from build123d import *

# Parameters (mm, degrees)
F0_R         = 7.935
F1_DEPTH     = 20
F2_DEPTH     = 12.7
F4_DEPTH     = 12.7
F6_T1_DEPTH  = 77.0257979591
F6_T3_DEPTH  = 76.8715237662
F6_T5_DEPTH  = 231
F6_T8_ANGLE  = 60.7302478015
F6_T12_DEPTH = 65.5200608313
F6_T17_DEPTH = 65.5200608313
F6_T20_ANGLE = 60.7302478015
F6_T22_ANGLE = 60.7302478015
F6_T26_DEPTH = 65.5200608313
F6_T31_DEPTH = 65.5200608313
F6_T34_ANGLE = 60.7302478015


# Not quite as in the source:
# - a fillet or chamfer that OpenCascade refuses, or shapes differently, is made with other operations: its cross-section is extruded or revolved along the edge and cut away or added


with BuildPart() as f1:
    # F0 (on Top) → F1 (new body)
    with BuildSketch(Plane.XY):
        with BuildLine():
            Line((98, 20), (-98, 20))
            ThreePointArc((-98, 20), (-99.4142135624, 19.4142135624), (-100, 18))
            Line((-100, 18), (-100, 2))
            ThreePointArc((-100, 2), (-99.4142135624, 0.5857864376), (-98, 0))
            Line((-98, 0), (-38.6284762338, 0))
            ThreePointArc((-38.6284762338, 0), (-33.5733896743, -1.3717846645), (-29.9052011587, -5.1107800249))
            Line((-29.9052011587, -5.1107800249), (-6.4271370964, -47))
            Line((-6.4271370964, -47), (-6.4271370964, -59.7))
            Line((-6.4271370964, -59.7), (6.2728629036, -59.7))
            Line((6.2728629036, -59.7), (6.2728629036, -47))
            Line((6.2728629036, -47), (29.7509269659, -5.1107800249))
            ThreePointArc((29.7509269659, -5.1107800249), (33.4191154814, -1.3717846645), (38.4742020409, 0))
            Line((38.4742020409, 0), (98, 0))
            ThreePointArc((98, 0), (99.4142135624, 0.5857864376), (100, 2))
            Line((100, 2), (100, 18))
            ThreePointArc((100, 18), (99.4142135624, 19.4142135624), (98, 20))
        make_face()
        Circle(F0_R, mode=Mode.SUBTRACT)
    extrude(amount=F1_DEPTH)

    # F2 (cut): a face of the model
    f2_faces = [f1.faces().sort_by_distance(p)[0] for p in [
        (-0.0771370964, -59.7, 10),
    ]]
    extrude(f2_faces, amount=-F2_DEPTH, mode=Mode.SUBTRACT)

    # F3 (on face) → F4 (join)
    with BuildSketch(Plane.XZ.offset(47)):
        with BuildLine():
            ThreePointArc((-6.4271370964, 10), (-0.0771370964, 3.65), (6.2728629036, 10))
            ThreePointArc((6.2728629036, 10), (-0.0771370964, 16.35), (-6.4271370964, 10))
        make_face()
    extrude(amount=F4_DEPTH)

    # F5: fillet of radius 6.0355339059 on 1 edges, made by hand

    # F5_s1 → F5_t2 (revolve, cut)
    with BuildSketch(Plane.XY.offset(10)):
        with BuildLine():
            ThreePointArc((-6.4271370964, -53.6644660941), (-4.6593701435, -57.932233047), (-0.3916031905, -59.7))
            Line((-0.3916031905, -59.7), (-6.4271370964, -59.7))
            Line((-6.4271370964, -59.7), (-6.4271370964, -53.6644660941))
        make_face()
    revolve(axis=Axis((-0.0771370964, -59.7, 10), (0, 1, 0)), mode=Mode.SUBTRACT)

    # F6: fillet of radius 7 on 14 edges, made by hand

    # F6_s2 → F6_t1 (cut)
    with BuildSketch(Plane.YZ.offset(38.4742020409)):
        with BuildLine():
            ThreePointArc((7, 0), (2.0502525317, 2.0502525317), (0, 7))
            Line((0, 7), (0, 0))
            Line((0, 0), (7, 0))
        make_face()
        with BuildLine():
            ThreePointArc((7, 20), (2.0502525317, 17.9497474683), (0, 13))
            Line((0, 13), (0, 20))
            Line((0, 20), (7, 20))
        make_face()
    extrude(amount=F6_T1_DEPTH, mode=Mode.SUBTRACT)

    # F6_s4 → F6_t3 (cut)
    with BuildSketch(Plane.YZ.offset(-115.5)):
        with BuildLine():
            ThreePointArc((7, 0), (2.0502525317, 2.0502525317), (0, 7))
            Line((0, 7), (0, 0))
            Line((0, 0), (7, 0))
        make_face()
        with BuildLine():
            ThreePointArc((7, 20), (2.0502525317, 17.9497474683), (0, 13))
            Line((0, 13), (0, 20))
            Line((0, 20), (7, 20))
        make_face()
    extrude(amount=F6_T3_DEPTH, mode=Mode.SUBTRACT)

    # F6_s6 → F6_t5 (cut)
    with BuildSketch(Plane.YZ.offset(-115.5)):
        with BuildLine():
            ThreePointArc((13, 0), (17.9497474683, 2.0502525317), (20, 7))
            Line((20, 7), (20, 0))
            Line((20, 0), (13, 0))
        make_face()
        with BuildLine():
            ThreePointArc((13, 20), (17.9497474683, 17.9497474683), (20, 13))
            Line((20, 13), (20, 20))
            Line((20, 20), (13, 20))
        make_face()
    extrude(amount=F6_T5_DEPTH, mode=Mode.SUBTRACT)

    # F6_s7 → F6_t8 (revolve, cut)
    with BuildSketch(Plane(origin=(4.9320537662, 8.7996985012, 0), x_dir=(0, 0, 1), z_dir=(-0.4889219975, -0.8723275075, 0))):
        with BuildLine():
            ThreePointArc((0, -21.4513247447), (2.0502525317, -26.401072213), (7, -28.4513247447))
            Line((7, -28.4513247447), (0, -28.4513247447))
            Line((0, -28.4513247447), (0, -21.4513247447))
        make_face()
    revolve(axis=Axis((38.4742020409, -10, 0), (0, 0, -1)), revolution_arc=F6_T8_ANGLE, mode=Mode.SUBTRACT)


with BuildPart() as f6_tool10:
    # F6_s11 → F6_t12 (new body)
    with BuildSketch(Plane(origin=(-27.1021452526, -48.3552528553, 0), x_dir=(0, 0, 1), z_dir=(0.4889219975, 0.8723275075, 0))):
        with BuildLine():
            ThreePointArc((7, 28.4513247447), (2.0502525317, 26.401072213), (0, 21.4513247447))
            Line((0, 21.4513247447), (0, 28.4513247447))
            Line((0, 28.4513247447), (7, 28.4513247447))
        make_face()
    extrude(amount=F6_T12_DEPTH)

    split(bisect_by=Plane.XZ.offset(47), keep=Keep.BOTTOM)


with BuildPart() as f1_1:
    add(f1.part)

    # F6_t9: cut F6_tool10
    add(f6_tool10.part, mode=Mode.SUBTRACT)


with BuildPart() as f6_tool15:
    # F6_s16 → F6_t17 (new body)
    with BuildSketch(Plane(origin=(-4.9689321973, 8.865496461, 0), x_dir=(0, 0, 1), z_dir=(0.4889219975, -0.8723275075, 0))):
        with BuildLine():
            ThreePointArc((7, 28.5859023668), (2.0502525317, 26.5356498351), (0, 21.5859023668))
            Line((0, 21.5859023668), (0, 28.5859023668))
            Line((0, 28.5859023668), (7, 28.5859023668))
        make_face()
    extrude(amount=F6_T17_DEPTH)

    split(bisect_by=Plane.XZ.offset(47), keep=Keep.BOTTOM)


with BuildPart() as f1_2:
    add(f1_1.part)

    # F6_t14: cut F6_tool15
    add(f6_tool15.part, mode=Mode.SUBTRACT)

    # F6_s19 → F6_t20 (revolve, cut)
    with BuildSketch(Plane.YZ.offset(-38.6284762338)):
        with BuildLine():
            ThreePointArc((7, 0), (2.0502525317, 2.0502525317), (0, 7))
            Line((0, 7), (0, 0))
            Line((0, 0), (7, 0))
        make_face()
    revolve(axis=Axis((-38.6284762338, -10, 0), (0, 0, -1)), revolution_arc=F6_T20_ANGLE, mode=Mode.SUBTRACT)

    # F6_s21 → F6_t22 (revolve, cut)
    with BuildSketch(Plane(origin=(4.9320537662, 8.7996985012, 0), x_dir=(0, 0, 1), z_dir=(-0.4889219975, -0.8723275075, 0))):
        with BuildLine():
            ThreePointArc((20, -21.4513247447), (17.9497474683, -26.401072213), (13, -28.4513247447))
            Line((13, -28.4513247447), (20, -28.4513247447))
            Line((20, -28.4513247447), (20, -21.4513247447))
        make_face()
    revolve(axis=Axis((38.4742020409, -10, 20), (0, 0, -1)), revolution_arc=F6_T22_ANGLE, mode=Mode.SUBTRACT)


with BuildPart() as f6_tool24:
    # F6_s25 → F6_t26 (new body)
    with BuildSketch(Plane(origin=(-27.1021452526, -48.3552528553, 0), x_dir=(0, 0, 1), z_dir=(0.4889219975, 0.8723275075, 0))):
        with BuildLine():
            ThreePointArc((13, 28.4513247447), (17.9497474683, 26.401072213), (20, 21.4513247447))
            Line((20, 21.4513247447), (20, 28.4513247447))
            Line((20, 28.4513247447), (13, 28.4513247447))
        make_face()
    extrude(amount=F6_T26_DEPTH)

    split(bisect_by=Plane.XZ.offset(47), keep=Keep.BOTTOM)


with BuildPart() as f1_3:
    add(f1_2.part)

    # F6_t23: cut F6_tool24
    add(f6_tool24.part, mode=Mode.SUBTRACT)


with BuildPart() as f6_tool29:
    # F6_s30 → F6_t31 (new body)
    with BuildSketch(Plane(origin=(-4.9689321973, 8.865496461, 0), x_dir=(0, 0, 1), z_dir=(0.4889219975, -0.8723275075, 0))):
        with BuildLine():
            ThreePointArc((20, 21.5859023668), (17.9497474683, 26.5356498351), (13, 28.5859023668))
            Line((13, 28.5859023668), (20, 28.5859023668))
            Line((20, 28.5859023668), (20, 21.5859023668))
        make_face()
    extrude(amount=F6_T31_DEPTH)

    split(bisect_by=Plane.XZ.offset(47), keep=Keep.BOTTOM)


with BuildPart() as f1_4:
    add(f1_3.part)

    # F6_t28: cut F6_tool29
    add(f6_tool29.part, mode=Mode.SUBTRACT)

    # F6_s33 → F6_t34 (revolve, cut)
    with BuildSketch(Plane.YZ.offset(-38.6284762338)):
        with BuildLine():
            ThreePointArc((7, 20), (2.0502525317, 17.9497474683), (0, 13))
            Line((0, 13), (0, 20))
            Line((0, 20), (7, 20))
        make_face()
    revolve(axis=Axis((-38.6284762338, -10, 20), (0, 0, -1)), revolution_arc=F6_T34_ANGLE, mode=Mode.SUBTRACT)


solid = f1_4.part
Build history of the part. All positions in model axes, mm. A direction names the side the tool comes from. Coordinates: 2 decimals unless noted, no trailing zeros. Write each loop counter-clockwise with the first axis right and the second up, starting at its lowest first coordinate (ties: lowest second). Pieces come first, ordered by that corner, then holes.
(1) Pin check, flat tips, straight feed: pin 1 Ø12 at (y, z) = (-32.5, 8) entering from +X; pin 2 Ø5 at (y, z) = (-30.5, 15) entering from -X; pin 3 Ø1.8 at (x, z) = (76.5, 9) entering from -Y; pin 4 Ø11 at (x, z) = (-0.5, 15) entering from -Y. Stop position of each tip, or through.
(2) Mould opens along X. For faces 1 (the flat face through (-8, -3, 20)), 2 (the flat face through (100, 10, 10)), 3 (the cylindrical face through (-1.72, -7.746, 9.86)) say: pulls with the +X half, pulls with the -X half, needs draft (parallel to the pull), parting line crosses it, or undercut.
(3) 3-axis set-ups, long thin cutter, end or side, ignore diameter. For faces 4 (the cylindrical face through (68.8, 2.1, 2)), 5 (the cylindrical face through (68.8, 2.1, 18)), 6 (the cylindrical face through (-1.45, -50.29, 3.8)), 7 (the flat face through (-69, 0, 10)), 8 (the flat face through (0, -47, 17)): which of +Z, -Z, +X, -X, +Y, -Y reach the whole face in a straight line?
(4) Drill centre lines: line 1 (Y direction, x = -6.5, z = 5); line 2 (Y direction, x = 0, z = 7.75) (3 decimals); line 3 (Z direction, x = -0.5, y = -52). Where is each one in solid material? Low to high.
(5) Cut at A-A on x = -40.5. List the corners of the cut face in (y, z), and give its area (3 significant figures).
Working result:
1. pin 1: stops at x = 17.76
1. pin 2: stops at x = -16.88
1. pin 3: stops at y = 0
1. pin 4: stops at y = -59.7
2. face 1: needs draft
2. face 2: pulls with the +X half
2. face 3: undercut
3. face 4: -Z, +X, -Y
3. face 5: +Z, +X, -Y
3. face 6: -Y
3. face 7: +Z, -Z, -X, -Y
3. face 8: +Z, -Y
4. line 1: y = -46.27 to -4.55, 4.55 to 19.71
4. line 2: y = -59.381 to -7.935, 7.935 to 20
4. line 3: z = 3.66 to 16.34
5. outline: (0, 7) arc R7 ccw to (7, 0) - (13, 0) arc R7 ccw to (20, 7) - (20, 13) arc R7 ccw to (13, 20) - (7, 20) arc R7 ccw to (0, 13) - close
5. area: 358 mm2
